from build123d import *

# Parameters (mm, degrees)
SALIENTE_EXTRUIR1_DEPTH = 100
CROQUIS2_W              = 100
CROQUIS2_H              = 100
SALIENTE_EXTRUIR2_DEPTH = 20
CROQUIS3_W              = 100
CROQUIS3_H              = 20
SALIENTE_EXTRUIR3_DEPTH = 1000
CROQUIS4_W              = 100
CROQUIS4_H              = 100
CROQUIS4_R              = 20
SALIENTE_EXTRUIR4_DEPTH = 10
CROQUIS7_R              = 20
CORTAR_EXTRUIR2_DEPTH   = 228.5


with BuildPart() as part:
    # Croquis1 → Saliente-Extruir1 (new body)
    with BuildSketch(Plane.XY):
        Polygon((0, 0), (50, 86.602540378), (150, 86.602540378), (200, 0), align=None)
    extrude(amount=SALIENTE_EXTRUIR1_DEPTH)

    # Croquis2 → Saliente-Extruir2 (add)
    with BuildSketch(Plane(origin=(0, 86.602540378, 0), x_dir=(1, 0, 0), z_dir=(0, 1, 0))):
        with Locations((100, -50)):
            Rectangle(CROQUIS2_W, CROQUIS2_H)
    extrude(amount=SALIENTE_EXTRUIR2_DEPTH)

    # Croquis3 → Saliente-Extruir3 (add)
    with BuildSketch(Plane.ZY.offset(-50)):
        with Locations((50, 96.602540378)):
            Rectangle(CROQUIS3_W, CROQUIS3_H)
    extrude(amount=SALIENTE_EXTRUIR3_DEPTH)

    # Croquis4 → Saliente-Extruir4 (add)
    with BuildSketch(Plane(origin=(0, 106.602540378, 0), x_dir=(1, 0, 0), z_dir=(0, 1, 0))):
        with Locations((100, -50)):
            Rectangle(CROQUIS4_W, CROQUIS4_H)
        with Locations(Location((100, -50, 0), (0, 0, 270))):
            Circle(CROQUIS4_R, mode=Mode.SUBTRACT)
    extrude(amount=SALIENTE_EXTRUIR4_DEPTH)

    # Croquis7 → Cortar-Extruir2 (cut, symmetric)
    with BuildSketch(Plane(origin=(0, 116.602540378, 0), x_dir=(1, 0, 0), z_dir=(0, 1, 0))):
        with Locations(Location((100, -50, 0), (0, 0, 270))):
            Circle(CROQUIS7_R)
    extrude(amount=CORTAR_EXTRUIR2_DEPTH, both=True, mode=Mode.SUBTRACT)


solid = part.part
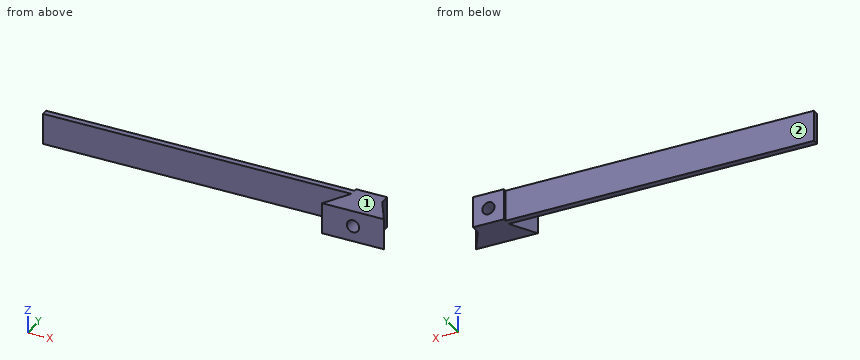
The listing builds one solid part. Answer for the finished solid, in the listing's coordinates (mm). Face numbers are marked on the shaded views. A direction names the side the tool comes from. Coordinates: 2 decimals unless noted, no trailing zeros. Order: outer loops, then holes, each group sorted by start corner. A loop starts at its lowest first (then second) coordinate and runs counter-clockwise, first axis right, second up. Notation, with made-up numbers: (52.25, 40.5) -> (99.25, 40.5) arc R19 ccw to (99.25, 63.5) -> close; hole circle Ø2 at (11.25, -26). An arc over 180 degrees is marked (long way). Answer in a Markdown table with one row per item. Add a question column.
Item 1: Find section A-A (z = 50). Write down the section's boundary in (x, y), then the cut area to 3 significant figures.
Item 2: Find the intervals of material crossed by L1, parallel to Y at x = -467, z = 25; L2, parallel to X at y = 54.5, z = 50; L3, parallel to X at y = 93, z = 50, in increasing order. Write a range as from..to.
Item 3: Find section C-C (y = 65.5). Write down the section's boundary in (x, z).
Item 4: Find section B-B (x = 100). Write down the section's boundary in (y, z).
Item 5: Which of the six approach directions +Z, -Z, +X, -X, +Y, -Y give full straight-line access (tool end or side, diameter ignored) to the marked faces 1 and 2?
Item 6: Each of these flat-tipped pins is pushed along its axis until it touches: P1, Ø1.5, axis at x = 9, z = 74.5, coming from the -Y side; P2, Ø3, axis at y = 112.5, z = 29.5, coming from the -X side; P3, Ø4, axis at y = 38, z = 28.5, coming from the -X side; P4, Ø1.5, axis at y = 53.5, z = 46, coming from the +X side. Where does it stop, or does it pass through?
Item 7: Find section D-D (x = -98). Write down the section's boundary in (y, z).
Result set:
| question | item | result |
|---|---|---|
| 1 | outline | (-950, 86.6) -> (50, 86.6) -> (0, 0) -> (80, 0) -> (80, 116.6) -> (50, 116.6) -> (50, 106.6) -> (-950, 106.6) -> close; (120, 0) -> (200, 0) -> (150, 86.6) -> (150, 116.6) -> (120, 116.6) -> close |
| 1 | area | 31,300 mm² |
| 2 | L1 | y = 86.6..106.6 |
| 2 | L2 | x = 31.47..80, 120..168.53 |
| 2 | L3 | x = -950..80, 120..150 |
| 3 | outline | (37.82, 0) -> (162.18, 0) -> (162.18, 100) -> (37.82, 100) -> close; hole circle Ø40 at (100, 50) |
| 4 | outline | (0, 0) -> (116.6, 0) -> (116.6, 30) -> (0, 30) -> close; (0, 70) -> (116.6, 70) -> (116.6, 100) -> (0, 100) -> close |
| 5 | face 1 | +Z, +X, -X, +Y, -Y |
| 5 | face 2 | +Z, -Z, -X, +Y |
| 6 | P1 | stops at y = 0 |
| 6 | P2 | stops at x = 50 |
| 6 | P3 | stops at x = 20.78 |
| 6 | P4 | stops at x = 169.54 |
| 7 | outline | (86.6, 0) -> (106.6, 0) -> (106.6, 100) -> (86.6, 100) -> close |
